```python
from build123d import *

# Parameters (mm, degrees)
ESQUISSE1_W             = 400
ESQUISSE1_H             = 180
BOSS_EXTRU_1_DEPTH      = 10
ESQUISSE2_W             = 80
ESQUISSE2_H             = 80
ENL_V_MAT_EXTRU_1_DEPTH = 10


with BuildPart() as part:
    # Esquisse1 → Boss.-Extru.1 (new body)
    with BuildSketch(Plane(origin=(0, 0, 0), x_dir=(1, 0, 0), z_dir=(0, 1, 0))):
        with Locations((-200, 90)):
            Rectangle(ESQUISSE1_W, ESQUISSE1_H)
    extrude(amount=BOSS_EXTRU_1_DEPTH)

    # Esquisse2 → Enlèv. mat.-Extru.1 (cut)
    with BuildSketch(Plane(origin=(0, 10, 0), x_dir=(1, 0, 0), z_dir=(0, 1, 0))):
        with Locations((-310, 80)):
            Rectangle(ESQUISSE2_W, ESQUISSE2_H)
        with Locations((-190, 80)):
            Rectangle(ESQUISSE2_W, ESQUISSE2_H)
        with Locations((-70, 80)):
            Rectangle(ESQUISSE2_W, ESQUISSE2_H)
    extrude(amount=-ENL_V_MAT_EXTRU_1_DEPTH, mode=Mode.SUBTRACT)


solid = part.part
```
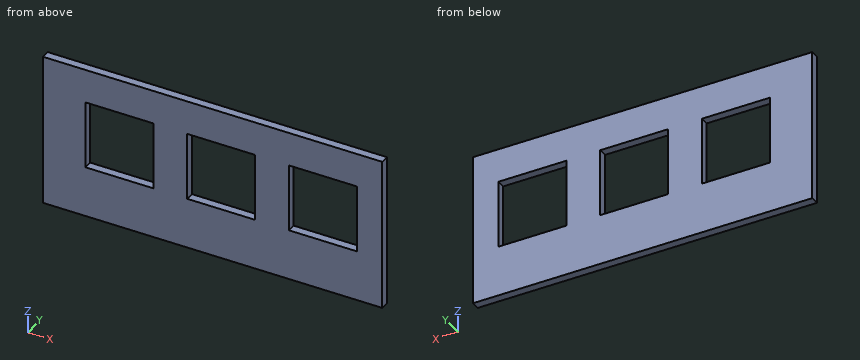
The listing builds one solid part. Answer for the finished solid, in the listing's coordinates (mm). Round coordinates to 2 decimals unless told otherwise and drop trailing zeros. Loops run counter-clockwise (first coordinate to the right, second up) from the corner with the lowest first, then second, coordinate; pieces in that order, holes last.
1) A cutting plane is placed at C-C on z = -73.5. Determine the outline of the cut face in (x, y), plus the area to 3 significant figures.
Outcome:
outline: (-400, 0) - (-350, 0) - (-350, 10) - (-400, 10) - close; (-270, 0) - (-230, 0) - (-230, 10) - (-270, 10) - close; (-150, 0) - (-110, 0) - (-110, 10) - (-150, 10) - close; (-30, 0) - (0, 0) - (0, 10) - (-30, 10) - close
area: 1,600 mm2
2) Consider line 1 (X direction, y = 6, z = -111.5); line 2 (Z direction, x = -157.5, y = 4.5). Determine where each line is inside the solid, lowest interval first.
Outcome:
line 1: x = -400 to -350, -270 to -230, -150 to -110, -30 to 0
line 2: z = -180 to -120, -40 to 0
3) Given P1, Ø12, axis at x = -280.5, z = -79.5, coming from the -Y side, flat-ended and moving along its own axis, determine where the tip first touches the part or whether it passes through.
Outcome:
P1: passes through
4) A cutting plane is placed at B-B on x = -60. Determine the outline of the cut face in (y, z), plus the area to 3 significant figures.
Outcome:
outline: (0, -180) - (10, -180) - (10, -120) - (0, -120) - close; (0, -40) - (10, -40) - (10, 0) - (0, 0) - close
area: 1,000 mm2
5) A cutting plane is placed at A-A on y = 5.25. Determine the outline of the cut face in (x, z), plus the area to 3 significant figures.
Outcome:
outline: (-400, -180) - (0, -180) - (0, 0) - (-400, 0) - close; hole (-350, -120) - (-270, -120) - (-270, -40) - (-350, -40) - close; hole (-230, -120) - (-150, -120) - (-150, -40) - (-230, -40) - close; hole (-110, -120) - (-30, -120) - (-30, -40) - (-110, -40) - close
area: 52,800 mm2
